Design review of the part built by this model. Coordinates are the model's own, in mm. A direction names the side the tool comes from. Give positions to 0.01 mm unless a question says otherwise; leave off trailing zeros. Write each loop counter-clockwise with the first axis right and the second up, starting at its lowest first coordinate (ties: lowest second). Pieces come first, ordered by that corner, then holes.
```python
from build123d import *

# Parameters (mm, degrees)
SKETCH1_R           = 5.08
SKETCH1_R_2         = 2.54
BOSS_EXTRUDE1_DEPTH = 0.762
CHAMFER2_SIZE       = 0.635
CHAMFER2_SIZE2      = 0.59214708
SKETCH3_R           = 5.08
SKETCH3_R_2         = 3.175
BOSS_EXTRUDE3_DEPTH = 0.508
BOSS_EXTRUDE4_START = 5.46608
SKETCH4_R           = 3.609397664
SKETCH4_R_2         = 2.54
BOSS_EXTRUDE4_DEPTH = 5.46608


with BuildPart() as part:
    # Sketch1 → Boss-Extrude1 (new body)
    with BuildSketch(Plane.XY):
        with Locations(Location((0, 0, 0), (0, 0, 180))):
            Circle(SKETCH1_R)
        with Locations(Location((0, 0, 0), (0, 0, 180))):
            Circle(SKETCH1_R_2, mode=Mode.SUBTRACT)
    extrude(amount=BOSS_EXTRUDE1_DEPTH)

    # Chamfer2
    chamfer2_edges = [part.edges().sort_by_distance(p)[0] for p in [
        (2.54, 0, 0.762),
    ]]
    chamfer2_side = [part.faces().sort_by_distance(p)[0] for p in [
        (4.936315902, 0, 0.762),
    ]]
    chamfer(chamfer2_edges, length=CHAMFER2_SIZE, length2=CHAMFER2_SIZE2, reference=chamfer2_side[0])

    # Sketch3 → Boss-Extrude3 (add)
    with BuildSketch(Plane.XY.offset(0.762)):
        with Locations(Location((0, 0, 0), (0, 0, 180))):
            Circle(SKETCH3_R)
        Circle(SKETCH3_R_2, mode=Mode.SUBTRACT)
    extrude(amount=BOSS_EXTRUDE3_DEPTH)

    # Sketch4 → Boss-Extrude4 (add)
    with BuildSketch(Plane(origin=(0, 0, 0), x_dir=(-1, 0, 0), z_dir=(0, 0, -1)).offset(BOSS_EXTRUDE4_START)):
        with Locations(Location((0, 0, 0), (0, 0, 180))):
            Circle(SKETCH4_R)
        Circle(SKETCH4_R_2, mode=Mode.SUBTRACT)
    extrude(amount=-BOSS_EXTRUDE4_DEPTH)


solid = part.part
```
(1) Consider section D-D, the plane x = 3.75. Give the boundary of the cut face in (y, z).
Resolved:
outline: (-3.43, 0) - (3.43, 0) - (3.43, 1.27) - (-3.43, 1.27) - close
(2) Clearance check with flat-ended pins moving along their axes: P1, Ø2, axis at y = 3.5, z = 0.5, coming from the +X side; P2, Ø5, axis at x = 0, y = 0, coming from the -Z side; P3, Ø1, axis at x = -2, z = -1.5, coming from the +Y side; P4, Ø1, axis at x = 2, z = -3.5, coming from the -Y side. State where each tip first meets the part, or that it passes through.
Resolved:
P1: stops at x = 4.42
P2: passes through
P3: stops at y = 3.28
P4: stops at y = -3.28
(3) Tool access review of faces 4 (the face through (1.94, -3.043, -2.771)), 5 (the face through (2, 2, -5.466)): name each direction out of +Z, -Z, +X, -X, +Y, -Y from which nothing blocks a thin tool from reaching the whole face with its end or side.
Resolved:
face 4: -Z
face 5: -Z, +X, -X, +Y, -Y
(4) To check wall thickness, follow L1, parallel to Y at x = 0, z = 0.15; L2, parallel to Y at x = 0, z = -3.25; L3, parallel to Z at x = 2.25, y = 3.5. State the ranges of each line that lie inside material, in increasing order.
Resolved:
L1: y = -5.08 to -2.54, 2.54 to 5.08
L2: y = -3.61 to -2.54, 2.54 to 3.61
L3: z = 0 to 1.27
(5) Consider section A-A, the plane x = 0. Give the boundary of the cut face in (y, z) (3 decimals), then the cut area to 3 significant figures.
Resolved:
outline: (-5.08, 0) - (-3.609, 0) - (-3.609, -5.466) - (-2.54, -5.466) - (-2.54, 0.17) - (-3.175, 0.762) - (-3.175, 1.27) - (-5.08, 1.27) - close; (2.54, -5.466) - (3.609, -5.466) - (3.609, 0) - (5.08, 0) - (5.08, 1.27) - (3.175, 1.27) - (3.175, 0.762) - (2.54, 0.17) - close
area: 17.1 mm2
(6) Consider section C-C, the plane z = -0.25. Give the boundary of the cut face in (x, y), then the cut area to 3 significant figures.
Resolved:
outline: circle Ø7.22 at (0, 0); hole circle Ø5.08 at (0, 0)
area: 20.7 mm2
(7) Mouldability with a two-part tool opening along Y and no side actions: class faces 1 (the face through (-2.2, 3.3, 0)), 2 (the face through (-0.69, -3.1, 1.01)), 3 (the face through (0.661, -5.037, 0.626)) as pulls with the +Y half, pulls with the -Y half, needs draft (parallel to the pull), parting line crosses it, or undercut.
Resolved:
face 1: needs draft
face 2: undercut
face 3: parting line crosses it
